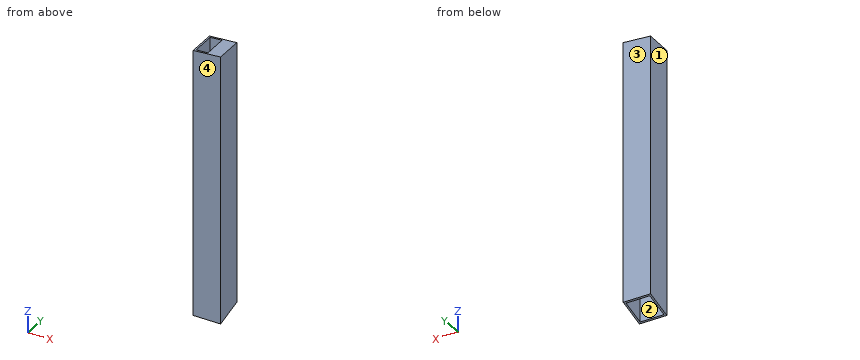
```python
from build123d import *

# Parameters (mm, degrees)
SKETCH1_W           = 25.4
SKETCH1_H           = 25.4
SKETCH1_W_2         = 22.098
SKETCH1_H_2         = 22.098
BOSS_EXTRUDE1_DEPTH = 250
SKETCH4_W           = 25.4
SKETCH4_H           = 25.4
BOSS_EXTRUDE2_DEPTH = 25.4
CUT_EXTRUDE1_DEPTH  = 165.021579309
CUT_EXTRUDE2_DEPTH  = 26.4


with BuildPart() as part:
    # Sketch1 → Boss-Extrude1 (new body)
    with BuildSketch(Plane.XY):
        Rectangle(SKETCH1_W, SKETCH1_H)
        Rectangle(SKETCH1_W_2, SKETCH1_H_2, mode=Mode.SUBTRACT)
    extrude(amount=BOSS_EXTRUDE1_DEPTH)

    # Sketch4 → Boss-Extrude2 (add)
    with BuildSketch(Plane.XY.offset(250)):
        Rectangle(SKETCH4_W, SKETCH4_H)
    extrude(amount=BOSS_EXTRUDE2_DEPTH)

    # Sketch5 → Cut-Extrude1 (cut, through all)
    with BuildSketch(Plane(origin=(-589.319373916, -151.321579309, 111.97168159), x_dir=(0, 0, -1), z_dir=(0, 1, 0))):
        Polygon((-140.246306665, -620.299815752), (-213.016787638, -571.728098704), (-135.810330154, -558.33893208), align=None)
    extrude(amount=CUT_EXTRUDE1_DEPTH, mode=Mode.SUBTRACT)

    # Sketch6 → Cut-Extrude2 (cut, through all)
    with BuildSketch(Plane(origin=(12.7, 0, 0), x_dir=(0, 0, -1), z_dir=(1, 0, 0))):
        Polygon((0, -12.7), (-11.495760494, 30.202762236), (0, 24.093064972), align=None)
    extrude(amount=-CUT_EXTRUDE2_DEPTH, mode=Mode.SUBTRACT)


solid = part.part
```
Source: CAD feature listing. Evaluate the final solid. Frame: model axes, mm. Face numbers are marked on the shaded views. Round coordinates to 2 decimals unless told otherwise and drop trailing zeros. Loops run counter-clockwise (first coordinate to the right, second up) from the corner with the lowest first, then second, coordinate; pieces in that order, holes last. Notation, with made-up numbers: (-36, -24) - (-3, -24) arc R27 ccw to (-3, 12) - close; hole circle Ø9 at (87.25, -10). An arc over 180 degrees is marked (long way). Use CSV: the item, a comma, the result in double quotes.
Q1. Ray query, line 1 along Y through (x, z) = (-5.5, 109); line 2 along Z through (x, y) = (9.5, 1.5). Return the intervals inside material, ascending.
Reported:
line 1,"-12.7 to -11.05, 11.05 to 12.7"
line 2,"250 to 250.68"
Q2. Section query B-B, the plane z = 203. Output: boundary loops of the cut face in (x, y), then the cut area to 3 significant figures.
Reported:
outline,"(-12.7, -12.7) - (12.7, -12.7) - (12.7, 12.7) - (-12.7, 12.7) - close; hole (-11.05, -11.05) - (11.05, -11.05) - (11.05, 11.05) - (-11.05, 11.05) - close"
area,"157 mm^2"
Q3. Section query A-A, the plane y = -8.75. Output: boundary loops of the cut face in (x, z).
Reported:
outline,"(-12.7, 1.06) - (-11.05, 1.06) - (-11.05, 249.21) - (-12.7, 249.09) - close; (0, 250) - (11.05, 250) - (11.05, 1.06) - (12.7, 1.06) - (12.7, 250.91) - close"
Q4. Pin query (flat end, axial travel): pin 1 Ø10 at (x, y) = (-1.5, -7.5) entering from -Z; pin 2 Ø3.5 at (x, y) = (7, 1) entering from -Z. Return the tip coordinate at first contact, or that it passes through.
Reported:
pin 1,"z = 0.05"
pin 2,"z = 250"
Q5. Section query D-D, the plane x = 4.5. Output: boundary loops of the cut face in (y, z).
Reported:
outline,"(-12.7, 0) - (-11.05, 0.44) - (-11.05, 250) - (11.05, 250) - (11.05, 6.36) - (12.7, 6.81) - (12.7, 250.32) - (-12.7, 250.32) - close"
Q6. Mould query, pull axis Y, two halves, no side actions, for the marked faces 1, 2, 3 and 4. Classes: pulls with the +Y half, pulls with the -Y half, needs draft (parallel to the pull), parting line crosses it, or undercut.
Reported:
face 1,"needs draft"
face 2,"undercut"
face 3,"pulls with the +Y half"
face 4,"pulls with the -Y half"
Q7. Section query C-C, the plane x = -5.5. Output: boundary loops of the cut face in (y, z).
Reported:
outline,"(-12.7, 0) - (-11.05, 0.44) - (-11.05, 249.61) - (-12.7, 249.61) - close; (11.05, 6.36) - (12.7, 6.81) - (12.7, 249.61) - (11.05, 249.61) - close"
